from build123d import *

# Parameters (mm, degrees)
BOSS_EXTRUDE1_DEPTH     = 25
CUT_EXTRUDE1_DEPTH      = 38.134889255
CUT_EXTRUDE1_DEPTH_BACK = 38.134889255
SKETCH2_R               = 12.8
SKETCH3_R               = 1.8
CUT_EXTRUDE2_DEPTH      = 16
SKETCH4_R               = 3.25
CUT_EXTRUDE3_DEPTH      = 5.6


with BuildPart() as part:
    # Sketch1 → Boss-Extrude1 (new, symmetric)
    with BuildSketch(Plane(origin=(0, 0, 0), x_dir=(0, 0, -1), z_dir=(1, 0, 0))):
        with BuildLine():
            Line((-19, -15), (19, -15))
            ThreePointArc((19, -15), (21.828427125, -13.828427125), (23, -11))
            Line((23, -11), (23, -4.6))
            ThreePointArc((23, -4.6), (21.828427125, -1.771572875), (19, -0.6))
            Line((19, -0.6), (-19, -0.6))
            ThreePointArc((-19, -0.6), (-21.828427125, -1.771572875), (-23, -4.6))
            Line((-23, -4.6), (-23, -11))
            ThreePointArc((-23, -11), (-21.828427125, -13.828427125), (-19, -15))
        make_face()
    extrude(amount=BOSS_EXTRUDE1_DEPTH, both=True)

    # Sketch2 → Cut-Extrude1 (cut, two sides: drawn at the far end of the back side and taken through both)
    with BuildSketch(Plane(origin=(0, 0, 0), x_dir=(0, 0, -1), z_dir=(1, 0, 0)).offset(-CUT_EXTRUDE1_DEPTH_BACK)):
        Circle(SKETCH2_R)
    extrude(amount=CUT_EXTRUDE1_DEPTH + CUT_EXTRUDE1_DEPTH_BACK, mode=Mode.SUBTRACT)

    # Sketch3 → Cut-Extrude2 (cut)
    with BuildSketch(Plane(origin=(0, -15, 0), x_dir=(1, 0, 0), z_dir=(0, 1, 0))):
        with Locations(Location((18, -17.5, 0), (0, 0, 236.442690238))):
            Circle(SKETCH3_R)
        with Locations(Location((18, 17.5, 0), (0, 0, 123.557309762))):
            Circle(SKETCH3_R)
        with Locations(Location((-18, -17.5, 0), (0, 0, 236.442690238))):
            Circle(SKETCH3_R)
        with Locations(Location((-18, 17.5, 0), (0, 0, 123.557309762))):
            Circle(SKETCH3_R)
    extrude(amount=CUT_EXTRUDE2_DEPTH, mode=Mode.SUBTRACT)

    # Sketch4 → Cut-Extrude3 (cut)
    with BuildSketch(Plane(origin=(0, -15, 0), x_dir=(1, 0, 0), z_dir=(0, 1, 0))):
        with Locations(Location((18, -17.5, 0), (0, 0, 207.48642625))):
            Circle(SKETCH4_R)
        with Locations(Location((18, 17.5, 0), (0, 0, 27.48642625))):
            Circle(SKETCH4_R)
        with Locations(Location((-18, -17.5, 0), (0, 0, 207.48642625))):
            Circle(SKETCH4_R)
        with Locations(Location((-18, 17.5, 0), (0, 0, 27.48642625))):
            Circle(SKETCH4_R)
    extrude(amount=CUT_EXTRUDE3_DEPTH, mode=Mode.SUBTRACT)


solid = part.part
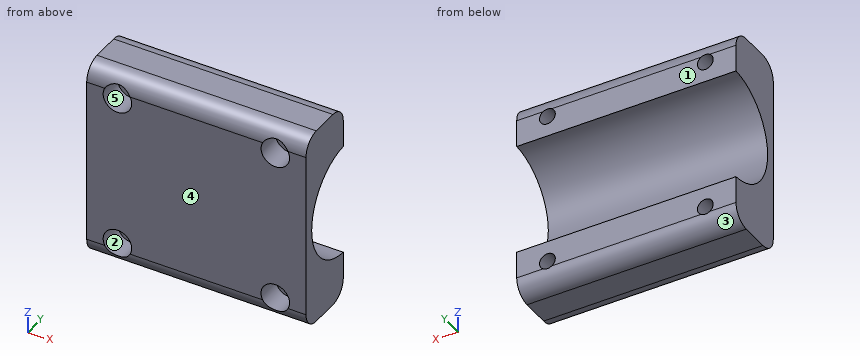
Could you check a few things on this model? Use its own coordinates, in mm. Face numbers are marked on the shaded views. A direction names the side the tool comes from. Coordinates: 2 decimals unless noted, no trailing zeros. Order: outer loops, then holes, each group sorted by start corner. A loop starts at its lowest first (then second) coordinate and runs counter-clockwise, first axis right, second up. Notation, with made-up numbers: (35.5, 40) - (92.5, 40) arc R24 ccw to (92.5, 59) - close; hole circle Ø6 at (86.25, 26.25). An arc over 180 degrees is marked (long way). Answer in a Markdown table with one row per item. Add a question column.
(1) Will these pins go through, and if not, where does the flat tip stop? pin 1 (2 mm diameter, centred on x = 18, z = -17.5, fed in from +Y); pin 2 (8 mm diameter, centred on x = 6.5, z = 5, fed in from +Y); pin 3 (3 mm diameter, centred on x = -19, z = -18, fed in from -Y).
(2) If we section it at A-A, the plane z = 17.5: Please give me the cut outline in (x, y), then the cut area to 3 significant figures.
(3) If we section it at B-B, the plane y = -2.25: Please give me the cut outline in (x, z).
(4) If we section it at D-D, the plane x = 6: Please give me the cut outline in (y, z), then the cut area to 3 significant figures.
(5) On a 3-axis mill with a long thin cutter (end or side, diameter ignored), from which of +Z, -Z, +X, -X, +Y, -Y can I reach the whole of each face in a straight line? I mean the marked faces 4 and 5. Say none if no direction works.
(6) If we mould it in two halves opening along Z, with no side actions, what happens to the marked faces 1, 2 and 3? For each: released by +Z, released by -Z, zero draft, split by the parting line, or undercut.
(7) I need wall thicknesses on L1, parallel to X at y = -3, z = -17.5; L2, parallel to X at y = -10.6, z = 17.5; L3, parallel to Z at x = -18, y = -11.3. Which ranges of each line are inside material? Lowest first, please.
(8) If we section it at C-C, the plane x = 18: Please give me the cut outline in (y, z), then the cut area to 3 significant figures.
Results are:
| question | item | result |
|---|---|---|
| 1 | pin 1 | passes through |
| 1 | pin 2 | stops at y = -9.1 |
| 1 | pin 3 | stops at y = -9.4 |
| 2 | outline | (-25, -15) - (-21.25, -15) - (-21.25, -9.4) - (-19.8, -9.4) - (-19.8, -0.6) - (-25, -0.6) - close; (-16.2, -9.4) - (-14.75, -9.4) - (-14.75, -15) - (14.75, -15) - (14.75, -9.4) - (16.2, -9.4) - (16.2, -0.6) - (-16.2, -0.6) - close; (19.8, -9.4) - (21.25, -9.4) - (21.25, -15) - (25, -15) - (25, -0.6) - (19.8, -0.6) - close |
| 2 | area | 584 mm2 |
| 3 | outline | (-25, -22.24) - (25, -22.24) - (25, -12.6) - (-25, -12.6) - close; (-25, 12.6) - (25, 12.6) - (25, 22.24) - (-25, 22.24) - close; hole circle Ø3.6 at (-18, -17.5); hole circle Ø3.6 at (-18, 17.5); hole circle Ø3.6 at (18, -17.5); hole circle Ø3.6 at (18, 17.5) |
| 4 | outline | (-15, -19) arc R4 ccw to (-11, -23) - (-4.6, -23) arc R4 ccw to (-0.6, -19) - (-0.6, -12.79) arc R12.8 cw to (-0.6, 12.79) - (-0.6, 19) arc R4 ccw to (-4.6, 23) - (-11, 23) arc R4 ccw to (-15, 19) - close |
| 4 | area | 407 mm2 |
| 5 | face 4 | +Z, -Z, +X, -X, -Y |
| 5 | face 5 | -Y |
| 6 | face 1 | zero draft |
| 6 | face 2 | undercut |
| 6 | face 3 | released by -Z |
| 7 | L1 | x = -25 to -19.8, -16.2 to 16.2, 19.8 to 25 |
| 7 | L2 | x = -25 to -21.25, -14.75 to 14.75, 21.25 to 25 |
| 7 | L3 | z = -22.99 to -20.75, -14.25 to -6.01, 6.01 to 14.25, 20.75 to 22.99 |
| 8 | outline | (-15, -14.25) - (-9.4, -14.25) - (-9.4, -15.7) - (-0.6, -15.7) - (-0.6, -12.79) arc R12.8 cw to (-0.6, 12.79) - (-0.6, 15.7) - (-9.4, 15.7) - (-9.4, 14.25) - (-15, 14.25) - close; (-14.6, -20.75) arc R4 ccw to (-11, -23) - (-4.6, -23) arc R4 ccw to (-0.61, -19.3) - (-9.4, -19.3) - (-9.4, -20.75) - close; (-14.6, 20.75) - (-9.4, 20.75) - (-9.4, 19.3) - (-0.61, 19.3) arc R4 ccw to (-4.6, 23) - (-11, 23) arc R4 ccw to start |
| 8 | area | 271 mm2 |
